Geometry check sheet. Reference: the model listing, model coordinates, mm. A direction names the side the tool comes from. Round coordinates to 2 decimals unless told otherwise and drop trailing zeros. Loops run counter-clockwise (first coordinate to the right, second up) from the corner with the lowest first, then second, coordinate; pieces in that order, holes last. Notation, with made-up numbers: (36.5, -36.75) -> (90.5, -36.75) arc R21 cw to (90.5, -28.75) -> close; hole circle Ø6 at (-9.75, 22.25). An arc over 180 degrees is marked (long way). Use one line per item in the form item = value.
from build123d import *

# Parameters (mm, degrees)
SKETCH1_R           = 60
SKETCH1_R_2         = 18
BOSS_EXTRUDE1_DEPTH = 7.5
CUT_EXTRUDE2_REACH  = 17
SKETCH3_R           = 2
SKETCH4_R           = 33
SKETCH4_R_2         = 31.5
SKETCH4_R_3         = 30
CUT_EXTRUDE3_DEPTH  = 3
SKETCH5_R           = 2.5
SKETCH6_R           = 3
CUT_EXTRUDE4_DEPTH  = 4
CUT_EXTRUDE5_REACH  = 17
SKETCH7_R           = 3


with BuildPart() as part:
    # Sketch1 → Boss-Extrude1 (new body, symmetric)
    with BuildSketch(Plane(origin=(0, 0, 0), x_dir=(0, 0, -1), z_dir=(1, 0, 0))):
        Circle(SKETCH1_R)
        Circle(SKETCH1_R_2, mode=Mode.SUBTRACT)
    extrude(amount=BOSS_EXTRUDE1_DEPTH, both=True)

    # Sketch3 → Cut-Extrude2 (cut, up to next)
    with BuildSketch(Plane(origin=(7.5, 0, 0), x_dir=(0, 0, -1), z_dir=(1, 0, 0)), mode=Mode.PRIVATE) as cut_extrude2_sk1:
        with Locations((0, 25)):
            Circle(SKETCH3_R)
    cut_extrude2_tool1 = extrude(cut_extrude2_sk1.sketch, amount=-CUT_EXTRUDE2_REACH, mode=Mode.PRIVATE) & part.part
    add(cut_extrude2_tool1.solids().sort_by_distance((7.5, 25, 0))[0], mode=Mode.SUBTRACT)
    # Sketch3 → Cut-Extrude2 (cut, up to next)
    with BuildSketch(Plane(origin=(7.5, 0, 0), x_dir=(0, 0, -1), z_dir=(1, 0, 0)), mode=Mode.PRIVATE) as cut_extrude2_sk2:
        with Locations((21.650635095, 12.5)):
            Circle(SKETCH3_R)
    cut_extrude2_tool2 = extrude(cut_extrude2_sk2.sketch, amount=-CUT_EXTRUDE2_REACH, mode=Mode.PRIVATE) & part.part
    add(cut_extrude2_tool2.solids().sort_by_distance((7.5, 12.5, -21.650635))[0], mode=Mode.SUBTRACT)
    # Sketch3 → Cut-Extrude2 (cut, up to next)
    with BuildSketch(Plane(origin=(7.5, 0, 0), x_dir=(0, 0, -1), z_dir=(1, 0, 0)), mode=Mode.PRIVATE) as cut_extrude2_sk3:
        with Locations((21.650635095, -12.5)):
            Circle(SKETCH3_R)
    cut_extrude2_tool3 = extrude(cut_extrude2_sk3.sketch, amount=-CUT_EXTRUDE2_REACH, mode=Mode.PRIVATE) & part.part
    add(cut_extrude2_tool3.solids().sort_by_distance((7.5, -12.5, -21.650635))[0], mode=Mode.SUBTRACT)
    # Sketch3 → Cut-Extrude2 (cut, up to next)
    with BuildSketch(Plane(origin=(7.5, 0, 0), x_dir=(0, 0, -1), z_dir=(1, 0, 0)), mode=Mode.PRIVATE) as cut_extrude2_sk4:
        with Locations((0, -25)):
            Circle(SKETCH3_R)
    cut_extrude2_tool4 = extrude(cut_extrude2_sk4.sketch, amount=-CUT_EXTRUDE2_REACH, mode=Mode.PRIVATE) & part.part
    add(cut_extrude2_tool4.solids().sort_by_distance((7.5, -25, 0))[0], mode=Mode.SUBTRACT)
    # Sketch3 → Cut-Extrude2 (cut, up to next)
    with BuildSketch(Plane(origin=(7.5, 0, 0), x_dir=(0, 0, -1), z_dir=(1, 0, 0)), mode=Mode.PRIVATE) as cut_extrude2_sk5:
        with Locations((-21.650635095, -12.5)):
            Circle(SKETCH3_R)
    cut_extrude2_tool5 = extrude(cut_extrude2_sk5.sketch, amount=-CUT_EXTRUDE2_REACH, mode=Mode.PRIVATE) & part.part
    add(cut_extrude2_tool5.solids().sort_by_distance((7.5, -12.5, 21.650635))[0], mode=Mode.SUBTRACT)
    # Sketch3 → Cut-Extrude2 (cut, up to next)
    with BuildSketch(Plane(origin=(7.5, 0, 0), x_dir=(0, 0, -1), z_dir=(1, 0, 0)), mode=Mode.PRIVATE) as cut_extrude2_sk6:
        with Locations((-21.650635095, 12.5)):
            Circle(SKETCH3_R)
    cut_extrude2_tool6 = extrude(cut_extrude2_sk6.sketch, amount=-CUT_EXTRUDE2_REACH, mode=Mode.PRIVATE) & part.part
    add(cut_extrude2_tool6.solids().sort_by_distance((7.5, 12.5, 21.650635))[0], mode=Mode.SUBTRACT)

    # Sketch4 → Cut-Extrude3 (cut)
    with BuildSketch(Plane.ZY.offset(7.5)):
        Circle(SKETCH4_R)
        Circle(SKETCH4_R_2, mode=Mode.SUBTRACT)
        Circle(SKETCH4_R_2)
        Circle(SKETCH4_R_3, mode=Mode.SUBTRACT)
    extrude(amount=-CUT_EXTRUDE3_DEPTH, mode=Mode.SUBTRACT)

    # Sketch5 → Cut-Revolve2 (revolve, cut)
    with BuildSketch(Plane.XY):
        with Locations((3.766886577, 60.013835775)):
            Circle(SKETCH5_R)
        with Locations((-3.766886577, 60.013835775)):
            Circle(SKETCH5_R)
    revolve(axis=Axis((7.5, 0, 0), (-1, 0, 0)), mode=Mode.SUBTRACT)

    # Sketch6 → Cut-Extrude4 (cut)
    with BuildSketch(Plane(origin=(7.5, 0, 0), x_dir=(0, 0, -1), z_dir=(1, 0, 0))):
        with Locations((0, 25)):
            Circle(SKETCH6_R)
        with Locations((21.650635095, 12.5)):
            Circle(SKETCH6_R)
        with Locations((21.650635095, -12.5)):
            Circle(SKETCH6_R)
        with Locations((0, -25)):
            Circle(SKETCH6_R)
        with Locations((-21.650635095, -12.5)):
            Circle(SKETCH6_R)
        with Locations((-21.650635095, 12.5)):
            Circle(SKETCH6_R)
    extrude(amount=-CUT_EXTRUDE4_DEPTH, mode=Mode.SUBTRACT)

    # Sketch7 → Cut-Extrude5 (cut, up to next)
    with BuildSketch(Plane.ZY.offset(7.5), mode=Mode.PRIVATE) as cut_extrude5_sk1:
        with Locations((-11, 19.052558883)):
            Circle(SKETCH7_R)
    cut_extrude5_tool1 = extrude(cut_extrude5_sk1.sketch, amount=-CUT_EXTRUDE5_REACH, mode=Mode.PRIVATE) & part.part
    add(cut_extrude5_tool1.solids().sort_by_distance((-7.5, 19.052559, -11))[0], mode=Mode.SUBTRACT)


solid = part.part
1. Section check B-B (z = 0). Count the separate pieces of the cut face and the enclosed holes in it, then the cut area to 3 significant figures.
Return value:
separate_pieces = 4
enclosed_holes = 0
area = 1,070 mm2
2. Tool access check on faces 1 (the cylindrical face through (-0.105, 17.847, 2.343)), 2 (the cylindrical face through (-6, -12.6, 30.5)), 3 (the cylindrical face through (5.53, 22.07, 0.65)). Record the directions out of +Z, -Z, +X, -X, +Y, -Y that give a thin tool (end or side, any length) a straight path to the whole face; none if there is none.
Return value:
face_1 = +X, -X
face_2 = -X
face_3 = +X
3. Section check A-A (y = 0). Record the boundary of the cut face in (x, z).
Return value:
outline = (-7.5, -60) -> (-6.27, -60) arc R2.5 cw to (-1.27, -60) -> (1.27, -60) arc R2.5 cw to (6.27, -60) -> (7.5, -60) -> (7.5, -18) -> (-7.5, -18) -> (-7.5, -30) -> (-4.5, -30) -> (-4.5, -33) -> (-7.5, -33) -> close; (-7.5, 18) -> (7.5, 18) -> (7.5, 60) -> (6.27, 60) arc R2.5 cw to (1.27, 60) -> (-1.27, 60) arc R2.5 cw to (-6.27, 60) -> (-7.5, 60) -> (-7.5, 33) -> (-4.5, 33) -> (-4.5, 30) -> (-7.5, 30) -> close
4. Material ranges on line 1 along Z through (x, y) = (3.25, -14); line 2 along Y through (x, z) = (-5, -3.5); line 3 along Z through (x, y) = (-5.5, -8.5), recorded low to high.
Return value:
line_1 = -55.84 to -22.97, -20.33 to -11.31, 11.31 to 20.33, 22.97 to 55.84
line_2 = -57.73 to -32.81, -29.8 to -17.66, 17.66 to 29.8, 32.81 to 57.73
line_3 = -57.59 to -31.89, -28.77 to -15.87, 15.87 to 28.77, 31.89 to 57.59
5. Gauge pin test, flat ends, axial feed: pin 1 (1.5 mm diameter, centred on x = 1.5, y = 31.5, fed in from -Z); pin 2 (3 mm diameter, centred on x = -4, y = -40.5, fed in from +Z); pin 3 (3 mm diameter, centred on y = 13, z = 21, fed in from +X). Record the tip position at first contact, or that the pin passes through.
Return value:
pin_1 = -51.5
pin_2 = 42.36
pin_3 = 3.5
6. Mould release check, pull along Z, two halves, no side actions. Record for faces 4 (the flat face through (-7.5, -13, -13)), 5 (the flat face through (3.5, -13, -24)), 6 (the cylindrical face through (0.02, 2.64, 59.94)): released by +Z, released by -Z, zero draft, split by the parting line, or undercut.
Return value:
face_4 = zero draft
face_5 = undercut
face_6 = split by the parting line
